CAD build for the part. Positions are in the model's coordinates, mm. Give positions to 0.01 mm unless a question says otherwise; leave off trailing zeros. Loops run counter-clockwise (first coordinate to the right, second up) from the corner with the lowest first, then second, coordinate; pieces in that order, holes last. Notation, with made-up numbers: (-36, 28) -> (16, 28) arc R9 cw to (16, 38) -> close; hole circle Ø10 at (13.5, 60.5). An arc over 180 degrees is marked (long way). Use one line per item in the form item = value.
```python
from build123d import *

# Parameters (mm, degrees)
MODEL_R         = 1.25
MODEL_R_2       = 1.65
MODEL_R_3       = 1.2
MODEL_R_4       = 1.5
EXTRUDE_1_DEPTH = 1.5


with BuildPart() as part:
    # Model → Бобышка-Вытянуть1 (new body)
    with BuildSketch(Plane.XY):
        with BuildLine():
            Line((-28.5, 0), (28.5, 0))
            ThreePointArc((28.5, 0), (29.207106781, 0.292893219), (29.5, 1))
            Line((29.5, 1), (29.5, 8))
            ThreePointArc((29.5, 8), (29.792893219, 8.707106781), (30.5, 9))
            Line((30.5, 9), (39, 9))
            ThreePointArc((39, 9), (39.707106781, 9.292893219), (40, 10))
            Line((40, 10), (40, 14))
            Line((40, 14), (40, 18))
            ThreePointArc((40, 18), (39.707106781, 18.707106781), (39, 19))
            Line((39, 19), (30.5, 19))
            ThreePointArc((30.5, 19), (29.792893219, 19.292893219), (29.5, 20))
            Line((29.5, 20), (29.5, 58))
            ThreePointArc((29.5, 58), (29.792893219, 58.707106781), (30.5, 59))
            Line((30.5, 59), (39, 59))
            ThreePointArc((39, 59), (39.707106781, 59.292893219), (40, 60))
            Line((40, 60), (40, 64))
            Line((40, 64), (40, 68))
            ThreePointArc((40, 68), (39.707106781, 68.707106781), (39, 69))
            Line((39, 69), (30.5, 69))
            ThreePointArc((30.5, 69), (29.792893219, 69.292893219), (29.5, 70))
            Line((29.5, 70), (29.5, 87))
            ThreePointArc((29.5, 87), (29.207106781, 87.707106781), (28.5, 88))
            Line((28.5, 88), (-28.5, 88))
            ThreePointArc((-28.5, 88), (-29.207106781, 87.707106781), (-29.5, 87))
            Line((-29.5, 87), (-29.5, 70))
            ThreePointArc((-29.5, 70), (-29.792893219, 69.292893219), (-30.5, 69))
            Line((-30.5, 69), (-39, 69))
            ThreePointArc((-39, 69), (-39.707106781, 68.707106781), (-40, 68))
            Line((-40, 68), (-40, 64))
            Line((-40, 64), (-40, 60))
            ThreePointArc((-40, 60), (-39.707106781, 59.292893219), (-39, 59))
            Line((-39, 59), (-30.5, 59))
            ThreePointArc((-30.5, 59), (-29.792893219, 58.707106781), (-29.5, 58))
            Line((-29.5, 58), (-29.5, 20))
            ThreePointArc((-29.5, 20), (-29.792893219, 19.292893219), (-30.5, 19))
            Line((-30.5, 19), (-39, 19))
            ThreePointArc((-39, 19), (-39.707106781, 18.707106781), (-40, 18))
            Line((-40, 18), (-40, 14))
            Line((-40, 14), (-40, 10))
            ThreePointArc((-40, 10), (-39.707106781, 9.292893219), (-39, 9))
            Line((-39, 9), (-30.5, 9))
            ThreePointArc((-30.5, 9), (-29.792893219, 8.707106781), (-29.5, 8))
            Line((-29.5, 8), (-29.5, 1))
            ThreePointArc((-29.5, 1), (-29.207106781, 0.292893219), (-28.5, 0))
        make_face()
        with Locations((-21, 9.75)):
            Circle(MODEL_R, mode=Mode.SUBTRACT)
        with Locations((-22.25, 83.75)):
            Circle(MODEL_R_2, mode=Mode.SUBTRACT)
        with Locations((-22.25, 44.25)):
            Circle(MODEL_R_2, mode=Mode.SUBTRACT)
        with Locations((-25.9, 33.75)):
            Circle(MODEL_R_3, mode=Mode.SUBTRACT)
        with Locations((-25.9, 25.75)):
            Circle(MODEL_R_3, mode=Mode.SUBTRACT)
        with Locations((-2.1, 33.75)):
            Circle(MODEL_R_3, mode=Mode.SUBTRACT)
        with Locations((-2.1, 25.75)):
            Circle(MODEL_R_3, mode=Mode.SUBTRACT)
        with Locations((2.1, 33.75)):
            Circle(MODEL_R_3, mode=Mode.SUBTRACT)
        with Locations((2.1, 25.75)):
            Circle(MODEL_R_3, mode=Mode.SUBTRACT)
        with Locations((-35, 64)):
            Circle(MODEL_R_4, mode=Mode.SUBTRACT)
        with Locations((-35, 14)):
            Circle(MODEL_R_4, mode=Mode.SUBTRACT)
        with Locations((21, 9.75)):
            Circle(MODEL_R, mode=Mode.SUBTRACT)
        with Locations((22.25, 83.75)):
            Circle(MODEL_R_2, mode=Mode.SUBTRACT)
        with Locations((22.25, 44.25)):
            Circle(MODEL_R_2, mode=Mode.SUBTRACT)
        with Locations((25.9, 33.75)):
            Circle(MODEL_R_3, mode=Mode.SUBTRACT)
        with Locations((25.9, 25.75)):
            Circle(MODEL_R_3, mode=Mode.SUBTRACT)
        with Locations((35, 64)):
            Circle(MODEL_R_4, mode=Mode.SUBTRACT)
        with Locations((35, 14)):
            Circle(MODEL_R_4, mode=Mode.SUBTRACT)
        with BuildLine():
            Line((-21.5, 37.75), (-21.5, 21.75))
            ThreePointArc((-21.5, 21.75), (-20.914213562, 20.335786438), (-19.5, 19.75))
            Line((-19.5, 19.75), (-8.5, 19.75))
            ThreePointArc((-8.5, 19.75), (-7.085786438, 20.335786438), (-6.5, 21.75))
            Line((-6.5, 21.75), (-6.5, 37.75))
            ThreePointArc((-6.5, 37.75), (-7.085786438, 39.164213562), (-8.5, 39.75))
            Line((-8.5, 39.75), (-19.5, 39.75))
            ThreePointArc((-19.5, 39.75), (-20.914213562, 39.164213562), (-21.5, 37.75))
        make_face(mode=Mode.SUBTRACT)
        with BuildLine():
            Line((19.5, 19.75), (8.5, 19.75))
            ThreePointArc((8.5, 19.75), (7.085786438, 20.335786438), (6.5, 21.75))
            Line((6.5, 21.75), (6.5, 37.75))
            ThreePointArc((6.5, 37.75), (7.085786438, 39.164213562), (8.5, 39.75))
            Line((8.5, 39.75), (19.5, 39.75))
            ThreePointArc((19.5, 39.75), (20.914213562, 39.164213562), (21.5, 37.75))
            Line((21.5, 37.75), (21.5, 21.75))
            ThreePointArc((21.5, 21.75), (20.914213562, 20.335786438), (19.5, 19.75))
        make_face(mode=Mode.SUBTRACT)
    extrude(amount=EXTRUDE_1_DEPTH)


solid = part.part
```
1. Cut at B-B, the plane y = 14. Write the cut outline in (x, z).
Result sheet:
outline = (-40, 0) -> (-36.5, 0) -> (-36.5, 1.5) -> (-40, 1.5) -> close; (-33.5, 0) -> (33.5, 0) -> (33.5, 1.5) -> (-33.5, 1.5) -> close; (36.5, 0) -> (40, 0) -> (40, 1.5) -> (36.5, 1.5) -> close
2. Cut at C-C, the plane x = 35. Write the cut outline in (y, z).
Result sheet:
outline = (9, 0) -> (12.5, 0) -> (12.5, 1.5) -> (9, 1.5) -> close; (15.5, 0) -> (19, 0) -> (19, 1.5) -> (15.5, 1.5) -> close; (59, 0) -> (62.5, 0) -> (62.5, 1.5) -> (59, 1.5) -> close; (65.5, 0) -> (69, 0) -> (69, 1.5) -> (65.5, 1.5) -> close
3. Cut at D-D, the plane y = 33.75. Write the cut outline in (x, z).
Result sheet:
outline = (-29.5, 0) -> (-27.1, 0) -> (-27.1, 1.5) -> (-29.5, 1.5) -> close; (-24.7, 0) -> (-21.5, 0) -> (-21.5, 1.5) -> (-24.7, 1.5) -> close; (-6.5, 0) -> (-3.3, 0) -> (-3.3, 1.5) -> (-6.5, 1.5) -> close; (-0.9, 0) -> (0.9, 0) -> (0.9, 1.5) -> (-0.9, 1.5) -> close; (3.3, 0) -> (6.5, 0) -> (6.5, 1.5) -> (3.3, 1.5) -> close; (21.5, 0) -> (24.7, 0) -> (24.7, 1.5) -> (21.5, 1.5) -> close; (27.1, 0) -> (29.5, 0) -> (29.5, 1.5) -> (27.1, 1.5) -> close
4. Cut at A-A, the plane x = 2.1. Write the cut outline in (y, z).
Result sheet:
outline = (0, 0) -> (24.55, 0) -> (24.55, 1.5) -> (0, 1.5) -> close; (26.95, 0) -> (32.55, 0) -> (32.55, 1.5) -> (26.95, 1.5) -> close; (34.95, 0) -> (88, 0) -> (88, 1.5) -> (34.95, 1.5) -> close
5. Mould opens along Y. For faces 1 (the flat face through (-1, 45, 0)), 2 (the cylindrical face through (1.84, 24.58, 0.74)) say: pulls with the +Y half, pulls with the -Y half, needs draft (parallel to the pull), parting line crosses it, or undercut.
Result sheet:
face_1 = needs draft
face_2 = undercut
6. Drill centre lines: line 1 (X direction, y = 64, z = 0.7); line 2 (X direction, y = 23.5, z = 0.2); line 3 (Y direction, x = -2.1, z = 0.75). Where is each one in solid material? Low to high.
Result sheet:
line_1 = -40 to -36.5, -33.5 to 33.5, 36.5 to 40
line_2 = -29.5 to -21.5, -6.5 to 6.5, 21.5 to 29.5
line_3 = 0 to 24.55, 26.95 to 32.55, 34.95 to 88
